Solid Edge part; units mm, degrees
sketch "Sketch1" plane through (0, 0, 0) normal (0, 0, 1) x (1, 0, 0)
  line L0 (88.2402, -52.6213) -> (-105.4348, -52.6213)
  line L1 (-105.4348, -52.6213) -> (-105.4348, 70.5687)
  line L2 (-105.4348, 70.5687) -> (88.2402, 70.5687)
  line L3 (88.2402, 70.5687) -> (88.2402, -52.6213)
extrude "Protrusion1" add sketch "Sketch1" against normal blind 1.5875
sketch "Sketch2" plane through (0, 0, 0) normal (0, 0, 1) x (1, 0, 0)
  circle A0 centre (-47.0216, -40.1665) radius 2.2225
  circle A1 centre (-46.5574, 54.8409) radius 2.2225
  circle A2 centre (52.6409, 54.1886) radius 2.2225
  circle A3 centre (52.5267, -40.6219) radius 2.2225
extrude "Protrusion2" add sketch "Sketch2" along normal up to vertex (4.2672 mm away)
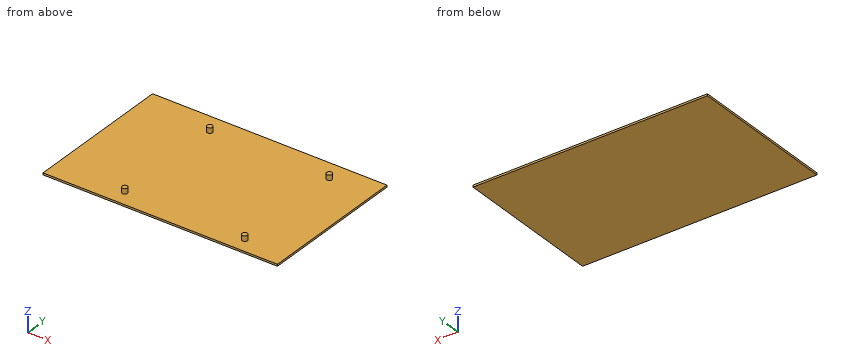
Design review of the part built by this model. Coordinates are the model's own, in mm. Round coordinates to 2 decimals unless told otherwise and drop trailing zeros. Write each loop counter-clockwise with the first axis right and the second up, starting at its lowest first coordinate (ties: lowest second). Pieces come first, ordered by that corner, then holes. Notation, with made-up numbers: (21, -16.75) - (30, -16.75) arc R27 ccw to (30, 11.25) - close; hole circle Ø3 at (0.5, -25). An arc over 180 degrees is marked (long way). Use a Markdown table: item, result. Add a question column.
1. Wall thickness on probe 1 along Z at (x, y) = (36.5, 22): over which ranges is the line inside the solid? List them lowest first.
2. We need section A-A (x = 31). State the section outline as (y, z) points.
3. We need section C-C (z = 3). State the section outline as (x, y) points (1 decimal), then the cut area to 3 significant figures.
4. We need section B-B (y = -33). State the section outline as (x, z) points.
5. Clearance check with a flat-ended pin moving along its axis: pin 1 (8 mm diameter, centred on x = -85.5, y = 6, fed in from +Z). State where the tip first meets the part, or that it passes through.
Output:
| question | item | result |
|---|---|---|
| 1 | probe 1 | z = -1.59 to 0 |
| 2 | outline | (-52.62, -1.59) - (70.57, -1.59) - (70.57, 0) - (-52.62, 0) - close |
| 3 | outline | circle Ø4.4 at (-47, -40.2); circle Ø4.4 at (-46.6, 54.8); circle Ø4.4 at (52.5, -40.6); circle Ø4.4 at (52.6, 54.2) |
| 3 | area | 62.1 mm2 |
| 4 | outline | (-105.43, -1.59) - (88.24, -1.59) - (88.24, 0) - (-105.43, 0) - close |
| 5 | pin 1 | stops at z = 0 |
